Design review of the part built by this model. Coordinates are the model's own, in mm. A direction names the side the tool comes from. Round coordinates to 2 decimals unless told otherwise and drop trailing zeros. Write each loop counter-clockwise with the first axis right and the second up, starting at its lowest first coordinate (ties: lowest second). Pieces come first, ordered by that corner, then holes.
from build123d import *

# Parameters (mm, degrees)
SKETCH1_R             = 3
BOSS_EXTRUDE1_DEPTH   = 10
BOSS_EXTRUDE1_2_DEPTH = 10
BOSS_EXTRUDE1_3_DEPTH = 10
BOSS_EXTRUDE1_4_DEPTH = 10
BOSS_EXTRUDE1_5_DEPTH = 10
BOSS_EXTRUDE1_6_DEPTH = 10
SKETCH2_R             = 25
BOSS_EXTRUDE2_DEPTH   = 7
SKETCH3_R             = 10
CUT_EXTRUDE1_DEPTH    = 40.230090492
SKETCH4_R             = 1.6
CUT_EXTRUDE2_DEPTH    = 10
SKETCH5_W             = 46.619491236
SKETCH5_H             = 46.698911153
CUT_EXTRUDE3_DEPTH    = 10
SKETCH6_R             = 3
CUT_EXTRUDE4_DEPTH    = 2


with BuildPart() as part:
    # Sketch1 → Boss-Extrude1 (new body)
    with BuildSketch(Plane(origin=(0, 0, 0), x_dir=(1, 0, 0), z_dir=(0, 1, 0))):
        with Locations(Location((0, 18, 0), (0, 0, 270))):
            Circle(SKETCH1_R)
    extrude(amount=BOSS_EXTRUDE1_DEPTH)



with BuildPart() as body_2:
    # Sketch1 → Boss-Extrude1 2 (new body)
    with BuildSketch(Plane(origin=(0, 0, 0), x_dir=(1, 0, 0), z_dir=(0, 1, 0))):
        with Locations(Location((15.588457268, 9, 0), (0, 0, 270))):
            Circle(SKETCH1_R)
    extrude(amount=BOSS_EXTRUDE1_2_DEPTH)


with BuildPart() as body_3:
    # Sketch1 → Boss-Extrude1 3 (new body)
    with BuildSketch(Plane(origin=(0, 0, 0), x_dir=(1, 0, 0), z_dir=(0, 1, 0))):
        with Locations(Location((15.588457268, -9, 0), (0, 0, 270))):
            Circle(SKETCH1_R)
    extrude(amount=BOSS_EXTRUDE1_3_DEPTH)


with BuildPart() as body_4:
    # Sketch1 → Boss-Extrude1 4 (new body)
    with BuildSketch(Plane(origin=(0, 0, 0), x_dir=(1, 0, 0), z_dir=(0, 1, 0))):
        with Locations(Location((0, -18, 0), (0, 0, 270))):
            Circle(SKETCH1_R)
    extrude(amount=BOSS_EXTRUDE1_4_DEPTH)


with BuildPart() as body_5:
    # Sketch1 → Boss-Extrude1 5 (new body)
    with BuildSketch(Plane(origin=(0, 0, 0), x_dir=(1, 0, 0), z_dir=(0, 1, 0))):
        with Locations(Location((-15.588457268, -9, 0), (0, 0, 270))):
            Circle(SKETCH1_R)
    extrude(amount=BOSS_EXTRUDE1_5_DEPTH)


with BuildPart() as body_6:
    # Sketch1 → Boss-Extrude1 6 (new body)
    with BuildSketch(Plane(origin=(0, 0, 0), x_dir=(1, 0, 0), z_dir=(0, 1, 0))):
        with Locations(Location((-15.588457268, 9, 0), (0, 0, 270))):
            Circle(SKETCH1_R)
    extrude(amount=BOSS_EXTRUDE1_6_DEPTH)


with BuildPart() as part_1:
    add(part.part)

    add(body_2.part)  # Boss-Extrude2 merges body 2

    add(body_3.part)  # Boss-Extrude2 merges body 3

    add(body_4.part)  # Boss-Extrude2 merges body 4

    add(body_5.part)  # Boss-Extrude2 merges body 5

    add(body_6.part)  # Boss-Extrude2 merges body 6
    # Sketch2 → Boss-Extrude2 (add)
    with BuildSketch(Plane(origin=(0, 10, 0), x_dir=(1, 0, 0), z_dir=(0, 1, 0))):
        with Locations(Location((0, 0, 0), (0, 0, 90))):
            Circle(SKETCH2_R)
    extrude(amount=BOSS_EXTRUDE2_DEPTH)

    # Sketch3 → Cut-Extrude1 (cut, through all)
    with BuildSketch(Plane(origin=(0, 17, 0), x_dir=(1, 0, 0), z_dir=(0, 1, 0))):
        with Locations(Location((0, 0, 0), (0, 0, 270))):
            Circle(SKETCH3_R)
    extrude(amount=-CUT_EXTRUDE1_DEPTH, mode=Mode.SUBTRACT)

    # Sketch4 → Cut-Extrude2 (cut)
    with BuildSketch(Plane(origin=(0, 17, 0), x_dir=(1, 0, 0), z_dir=(0, 1, 0))):
        with Locations(Location((0, 18, 0), (0, 0, 270))):
            Circle(SKETCH4_R)
        with Locations(Location((15.588457268, 9, 0), (0, 0, 270))):
            Circle(SKETCH4_R)
        with Locations(Location((15.588457268, -9, 0), (0, 0, 270))):
            Circle(SKETCH4_R)
        with Locations(Location((0, -18, 0), (0, 0, 270))):
            Circle(SKETCH4_R)
        with Locations(Location((-15.588457268, -9, 0), (0, 0, 270))):
            Circle(SKETCH4_R)
        with Locations(Location((-15.588457268, 9, 0), (0, 0, 270))):
            Circle(SKETCH4_R)
    extrude(amount=-CUT_EXTRUDE2_DEPTH, mode=Mode.SUBTRACT)

    # Sketch5 → Cut-Extrude3 (cut)
    with BuildSketch(Plane.XZ):
        with Locations((3.295926552, -0.079419917)):
            Rectangle(SKETCH5_W, SKETCH5_H)
    extrude(amount=-CUT_EXTRUDE3_DEPTH, mode=Mode.SUBTRACT)

    # Sketch6 → Cut-Extrude4 (cut)
    with BuildSketch(Plane(origin=(0, 10, 0), x_dir=(-1, 0, 0), z_dir=(0, -1, 0))):
        with Locations(Location((0, -18, 0), (0, 0, 90))):
            Circle(SKETCH6_R)
        with Locations(Location((15.588457268, 9, 0), (0, 0, 90))):
            Circle(SKETCH6_R)
        with Locations(Location((-15.588457268, 9, 0), (0, 0, 90))):
            Circle(SKETCH6_R)
    extrude(amount=-CUT_EXTRUDE4_DEPTH, mode=Mode.SUBTRACT)


solid = part_1.part
1) For P1, Ø5.5, axis at x = 0, z = 18, coming from the -Y side; P2, Ø3, axis at x = 10, y = 15.5, coming from the +Z side; P3, Ø1, axis at x = 16, y = 15, coming from the +Z side, all flat-tipped, find the tip position at first contact; note any pin that passes through.
2) The part is to be moulded in two halves that separate along Z. For faces 3 (the face through (11, 10, 0)), 4 (the face through (-7.509, 13.451, -23.846)), 5 (the face through (-13.059, 10.986, -10.613)), say which applies: pulls with the +Z half, pulls with the -Z half, needs draft (parallel to the pull), parting line crosses it, or undercut.
3) Add section A-A on z = 0. State the section outline as (x, y) points, and give its area (3 significant figures).
4) For faces 1 (the face through (18.12, 10.99, -10.61)), 2 (the face through (0, 17, -11)), list the 3-axis set-ups (+Z, -Z, +X, -X, +Y, -Y) from which the entire face can be reached by the end or side of a thin tool; tool diameter is ignored.
5) Add section D-D on z = -18. State the section outline as (x, y) points.
6) For line 1 along X through (y, z) = (11.4, -9); line 2 along X through (y, z) = (15, 9); line 3 along Z through (x, y) = (-16.5, 15.75), list the stretches that pass through material, from the lowest coordinate up.
7) Add section B-B on z = -9. State the section outline as (x, y) points.
8) Add section C-C on y = 13.25. State the section outline as (x, z) points, and give its area (3 significant figures).
Computed:
1. P1: stops at y = 12
1. P2: stops at z = 23.51
1. P3: stops at z = 19.62
2. face 3: needs draft
2. face 4: parting line crosses it
2. face 5: undercut
3. outline: (-25, 10) - (-10, 10) - (-10, 17) - (-25, 17) - close; (10, 10) - (25, 10) - (25, 17) - (10, 17) - close
3. area: 210 mm2
4. face 1: -Y
4. face 2: +Z, -Z, +X, -X, +Y
5. outline: (-17.35, 10) - (-1.6, 10) - (-1.6, 17) - (-17.35, 17) - close; (1.6, 10) - (17.35, 10) - (17.35, 17) - (1.6, 17) - close
6. line 1: x = -23.32 to -18.59, -12.59 to -4.36, 4.36 to 12.59, 18.59 to 23.32
6. line 2: x = -23.32 to -17.19, -13.99 to -4.36, 4.36 to 13.99, 17.19 to 23.32
6. line 3: z = -18.78 to -10.31, -7.69 to 7.69, 10.31 to 18.78
7. outline: (-23.32, 10) - (-18.59, 10) - (-18.59, 12) - (-17.19, 12) - (-17.19, 17) - (-23.32, 17) - close; (-13.99, 12) - (-12.59, 12) - (-12.59, 10) - (-4.36, 10) - (-4.36, 17) - (-13.99, 17) - close; (4.36, 10) - (12.59, 10) - (12.59, 12) - (13.99, 12) - (13.99, 17) - (4.36, 17) - close; (17.19, 12) - (18.59, 12) - (18.59, 10) - (23.32, 10) - (23.32, 17) - (17.19, 17) - close
8. outline: circle Ø50 at (0, 0); hole circle Ø3.2 at (-15.59, -9); hole circle Ø3.2 at (-15.59, 9); hole circle Ø20 at (0, 0); hole circle Ø3.2 at (0, -18); hole circle Ø3.2 at (0, 18); hole circle Ø3.2 at (15.59, -9); hole circle Ø3.2 at (15.59, 9)
8. area: 1,600 mm2
